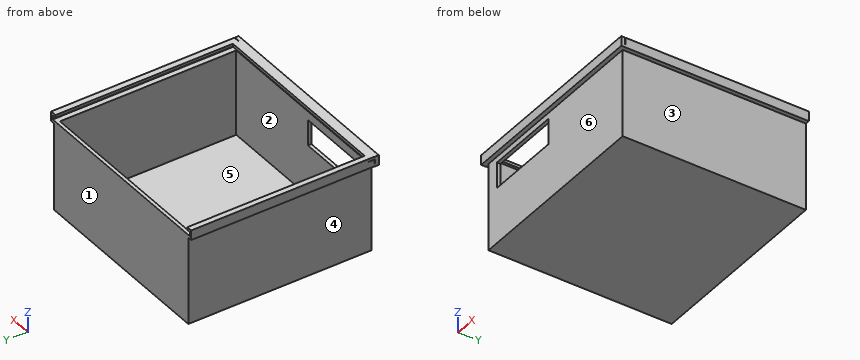
```python
from build123d import *

# Parameters (mm, degrees)
F0_W      = 140
F0_H      = 130
F1_DEPTH  = 65
F2_W      = 138
F2_H      = 128
F3_DEPTH  = 63
F4_W      = 60
F4_H      = 20
F5_DEPTH  = 25
F7_W      = 130
F7_H      = 2.0862916112
F8_DEPTH  = 3
F9_W      = 1.5
F9_H      = 130
F10_DEPTH = 5
F11_W     = 130
F11_H     = 2
F12_DEPTH = 3
F13_W     = 130
F13_H     = 2
F14_DEPTH = 3
F15_W     = 1
F15_H     = 130
F16_DEPTH = 5
F17_W     = 130
F17_H     = 2
F18_DEPTH = 3
F19_DEPTH = 1.5
F20_DEPTH = 1.5
F21_DEPTH = 1.5
F22_DEPTH = 1.5
F23_DEPTH = 1.5
F25_DEPTH = 3
F26_W     = 80.1923086047
F26_H     = 2.75
F27_DEPTH = 5
F28_W     = 75.8964964747
F28_H     = 2.1470558643
F29_DEPTH = 4.5
F30_W     = 59.895
F30_H     = 4
F31_DEPTH = 3
F32_DEPTH = 62
F33_W     = 53.8761485368
F33_H     = 18.5779780149
F34_DEPTH = 3
F35_DEPTH = 4


with BuildPart() as f1:
    # F0 (on Top) → F1 (new body)
    with BuildSketch(Plane.XY):
        Rectangle(F0_W, F0_H)
    extrude(amount=F1_DEPTH)

    # F2 (on face) → F3 (cut)
    with BuildSketch(Plane.XY.offset(65)):
        Rectangle(F2_W, F2_H)
    extrude(amount=-F3_DEPTH, mode=Mode.SUBTRACT)

    # F4 (on face) → F5 (cut)
    with BuildSketch(Plane.XZ.offset(65)):
        with Locations((-37.1923086047, 55)):
            Rectangle(F4_W, F4_H)
    extrude(amount=-F5_DEPTH, mode=Mode.SUBTRACT)

    # F7 (on face) → F8 (join)
    with BuildSketch(Plane.YZ.offset(70)):
        with Locations((0, 63.9568541944)):
            Rectangle(F7_W, F7_H)
    extrude(amount=F8_DEPTH)

    # F9 (on face) → F10 (join)
    with BuildSketch(Plane.XY.offset(65)):
        with Locations((72.25, 0)):
            Rectangle(F9_W, F9_H)
    extrude(amount=F10_DEPTH)

    # F11 (on face) → F12 (join)
    with BuildSketch(Plane(origin=(71.5, 0, 0), x_dir=(0, -1, 0), z_dir=(-1, 0, 0))):
        with Locations((0, 69)):
            Rectangle(F11_W, F11_H)
    extrude(amount=F12_DEPTH)

    # F13 (on face) → F14 (join)
    with BuildSketch(Plane(origin=(-70, 0, 0), x_dir=(0, -1, 0), z_dir=(-1, 0, 0))):
        with Locations((0, 64)):
            Rectangle(F13_W, F13_H)
    extrude(amount=F14_DEPTH)

    # F15 (on face) → F16 (join)
    with BuildSketch(Plane.XY.offset(65)):
        with Locations((-72.5, 0)):
            Rectangle(F15_W, F15_H)
    extrude(amount=F16_DEPTH)

    # F17 (on face) → F18 (join)
    with BuildSketch(Plane.YZ.offset(-72)):
        with Locations((0, 69)):
            Rectangle(F17_W, F17_H)
    extrude(amount=F18_DEPTH)

    # F19 (add): a face of the model
    f19_faces = [f1.faces().sort_by_distance(p)[0] for p in [
        (5.6478539393, -65, 29.2570369854),
    ]]
    extrude(f19_faces, amount=F19_DEPTH)

    # F20 (add): a face of the model
    f20_faces = [f1.faces().sort_by_distance(p)[0] for p in [
        (0, 64, 33.5),
    ]]
    extrude(f20_faces, amount=F20_DEPTH)

    # F21 (add): a face of the model
    f21_faces = [f1.faces().sort_by_distance(p)[0] for p in [
        (-69, -0.75, 33.5),
    ]]
    extrude(f21_faces, amount=F21_DEPTH)

    # F22 (add): a face of the model
    f22_faces = [f1.faces().sort_by_distance(p)[0] for p in [
        (0.75, -0.75, 2),
    ]]
    extrude(f22_faces, amount=F22_DEPTH)

    # F23 (add): a face of the model
    f23_faces = [f1.faces().sort_by_distance(p)[0] for p in [
        (69, -0.75, 34.25),
    ]]
    extrude(f23_faces, amount=F23_DEPTH)

    # F24 (on face) → F25 (join)
    with BuildSketch(Plane.XZ.offset(66.5)):
        Polygon((70, 62.9137083888), (73, 62.9137083888), (73, 65), (71.5, 65), (-7.1923086047, 65), (-7.1923086047, 62.9137083888), align=None)
    extrude(amount=F25_DEPTH)

    # F26 (on face) → F27 (join)
    with BuildSketch(Plane.XY.offset(65)):
        with Locations((32.9038456976, -68.125)):
            Rectangle(F26_W, F26_H)
    extrude(amount=F27_DEPTH)

    # F28 (on face) → F29 (join)
    with BuildSketch(Plane(origin=(0, -66.75, 0), x_dir=(-1, 0, 0), z_dir=(0, 1, 0))):
        with Locations((-30.7559396327, 68.9264720678)):
            Rectangle(F28_W, F28_H)
    extrude(amount=F29_DEPTH)

    # F30 (on face) → F31 (cut)
    with BuildSketch(Plane.XZ.offset(66.5)):
        with Locations((-37.1398086047, 43)):
            Rectangle(F30_W, F30_H)
    extrude(amount=-F31_DEPTH, mode=Mode.SUBTRACT)

    # F32 (add): a face of the model
    f32_faces = [f1.faces().sort_by_distance(p)[0] for p in [
        (-7.1923086047, -65.8019850182, 57.704218208),
    ]]
    extrude(f32_faces, amount=F32_DEPTH)

    # F33 (on face) → F34 (cut)
    with BuildSketch(Plane.XZ.offset(66.5)):
        with Locations((-34.1628445312, 49.4380742311)):
            Rectangle(F33_W, F33_H)
    extrude(amount=-F34_DEPTH, mode=Mode.SUBTRACT)

    # F35 (add): a face of the model
    f35_faces = [f1.faces().sort_by_distance(p)[0] for p in [
        (-69.1923086047, -67.9393083677, 66.5012630043),
    ]]
    extrude(f35_faces, amount=F35_DEPTH)


solid = f1.part
```
Model file for the job. Use its own axes, mm. Face numbers are marked on the shaded views. A direction names the side the tool comes from. Give positions to 0.01 mm unless a question says otherwise; leave off trailing zeros. Loops run counter-clockwise (first coordinate to the right, second up) from the corner with the lowest first, then second, coordinate; pieces in that order, holes last. Notation, with made-up numbers: (-5, 18.5) - (28, 18.5) arc R30 cw to (28, 51.5) - close; hole circle Ø1 at (31, 27). An arc over 180 degrees is marked (long way). One line per item, written item: value. Start each with the question number.
1. Slice it at D-D (x = 63.5). List the corners of the cut face in (y, z), plus the area to 3 significant figures.
2. Slice it at C-C (y = 11). List the corners of the cut face in (x, z).
3. Pull direction X, two halves, no side cores. Call the marked faces 4, 5 and 6: pulls with the +X half, pulls with the -X half, needs draft (parallel to the pull), parting line crosses it, or undercut.
4. Pin check, flat tips, straight feed: pin 1 (2.5 mm diameter, centred on x = -71.5, y = -17.5, fed in from -Z); pin 2 (3 mm diameter, centred on x = 25, y = -36, fed in from +Z); pin 3 (6 mm diameter, centred on y = -23.5, z = 53.5, fed in from +X). Stop position of each tip, or through.
5. Probe L1, parallel to Y at x = -39, z = 17; L2, parallel to X at y = -42.5, z = 51.5; L3, parallel to Y at x = 12.5, z = 64. List the from-to ranges inside material, lowest first. Write a range as from..to.
6. Slice it at A-A (z = 36.5). List the corners of the cut face in (x, y).
7. Which spindle directions (+Z, -Z, +X, -X, +Y, -Y) get a long thin tool onto all of the face, cutting with end or side? Do the marked faces 1, 2 and 3. Say none if no direction does.
8. Slice it at B-B (x = -10). List the corners of the cut face in (y, z), plus the area to 3 significant figures.
Solution:
1. outline: (-69.5, 62.91) - (-66.5, 62.91) - (-66.5, 0) - (65, 0) - (65, 65) - (62.5, 65) - (62.5, 3.5) - (-64, 3.5) - (-64, 65) - (-66.75, 65) - (-66.75, 67.85) - (-62.25, 67.85) - (-62.25, 70) - (-69.5, 70) - close
1. area: 797 mm^2
2. outline: (-73, 63) - (-70, 63) - (-70, 0) - (70, 0) - (70, 62.91) - (73, 62.91) - (73, 70) - (68.5, 70) - (68.5, 68) - (71.5, 68) - (71.5, 65) - (67.5, 65) - (67.5, 3.5) - (-67.5, 3.5) - (-67.5, 65) - (-72, 65) - (-72, 68) - (-69, 68) - (-69, 70) - (-73, 70) - close
3. face 4: pulls with the -X half
3. face 5: undercut
3. face 6: needs draft
4. pin 1: stops at z = 63
4. pin 2: stops at z = 3.5
4. pin 3: stops at x = 70
5. L1: y = -66.5..-64, 62.5..65
5. L2: x = -70..-67.5, 67.5..70
5. L3: y = -69.5..-64, 62.5..65
6. outline: (-70, -66.5) - (70, -66.5) - (70, 65) - (-70, 65) - close; hole (-67.5, -64) - (67.5, -64) - (67.5, 62.5) - (-67.5, 62.5) - close
7. face 1: +Z, -Z, +X, -X, +Y
7. face 2: none
7. face 3: -Z, +X, +Y, -Y
8. outline: (-69.5, 62.91) - (-66.5, 62.91) - (-66.5, 58.73) - (-64, 58.73) - (-64, 65) - (-66.75, 65) - (-66.75, 67.85) - (-62.25, 67.85) - (-62.25, 70) - (-69.5, 70) - close; (-66.5, 0) - (65, 0) - (65, 65) - (62.5, 65) - (62.5, 3.5) - (-64, 3.5) - (-64, 40.15) - (-66.5, 40.15) - close
8. area: 751 mm^2
